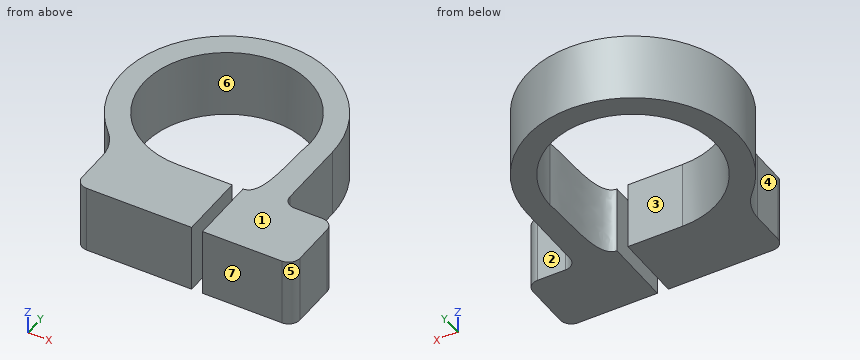
from build123d import *

# Parameters (mm, degrees)
F1_DEPTH = 9.525


with BuildPart() as f1:
    # F0 (on Top) → F1 (new body)
    with BuildSketch(Plane.XY):
        with BuildLine():
            ThreePointArc((0, -11.58875), (-8.194484, 8.194484), (11.58875, 0))
            add(Edge.make_bspline(
                [(9.147086, -11.58875), (12.021219, -11.58875), (11.099955, -3.330184), (11.58875, 0)],
                knots=[0, 0, 0, 0, 11.843177, 11.843177, 11.843177, 11.843177], degree=3))
            Line((9.147086, -11.58875), (9.147086, -21.11375))
            Line((9.147086, -21.11375), (20.259586, -21.11375))
            ThreePointArc((20.259586, -21.11375), (21.382118, -20.648782), (21.847086, -19.52625))
            Line((21.847086, -19.52625), (21.847086, -13.17625))
            ThreePointArc((21.847086, -13.17625), (21.382118, -12.053718), (20.259586, -11.58875))
            Line((20.259586, -11.58875), (16.35125, -11.58875))
            ThreePointArc((16.35125, -11.58875), (15.228718, -11.123782), (14.76375, -10.00125))
            Line((14.76375, -10.00125), (14.76375, 0))
            ThreePointArc((14.76375, 0), (-5.649843, 13.639926), (-10.439548, -10.439548))
            ThreePointArc((-10.439548, -10.439548), (-9.113907, -12.423509), (-8.648405, -14.76375))
            Line((-8.648405, -14.76375), (-8.648405, -19.52625))
            ThreePointArc((-8.648405, -19.52625), (-8.183437, -20.648782), (-7.060905, -21.11375))
            Line((-7.060905, -21.11375), (7.620076, -21.11375))
            Line((7.620076, -21.11375), (7.620076, -11.58875))
            Line((7.620076, -11.58875), (0, -11.58875))
        make_face()
    extrude(amount=F1_DEPTH)


solid = f1.part
Input: part model. Units: mm. Frame: model coordinates. Face numbers are marked on the shaded views. A direction names the side the tool comes from. Coordinates: 2 decimals unless noted, no trailing zeros. Loops run counter-clockwise (first coordinate to the right, second up) from the corner with the lowest first, then second, coordinate; pieces in that order, holes last.
(1) Section A-A on y = -17.5. Return the cut outline in (x, z) (3 decimals).
(2) Material intervals for probe 1 along Y at (x, z) = (0, 4.75); probe 2 along Y at (x, z) = (18, 3); probe 3 along Y at (x, z) = (5, 8), sorted ascending.
(3) Set-up query: the marked faces 1, 2, 3 and 4. Return all of +Z, -Z, +X, -X, +Y, -Y with unobstructed straight access to the full face (end or side cutting, diameter ignored); none if empty.
(4) First-contact query: pin 1 Ø1.5 at (x, z) = (0.5, 2) entering from +Y; pin 2 Ø2 at (y, z) = (11, 3) entering from +X; pin 3 Ø1 at (x, y) = (15, 3) entering from +Z; pin 4 Ø3 at (x, z) = (7.5, 5) entering from +Y. Flat tips, straight axial feed; report the tip coordinate or a pass-through.
(5) Section B-B on x = 4. Return the cut outline in (y, z) (3 decimals).
(6) Pull-direction query (X, two-part tool) for the marked faces 5, 6 and 7; classes: released by +X, released by -X, zero draft, split by the parting line, or undercut.
Data:
1. outline: (-8.648, 0) - (7.62, 0) - (7.62, 9.525) - (-8.648, 9.525) - close; (9.147, 0) - (21.847, 0) - (21.847, 9.525) - (9.147, 9.525) - close
2. probe 1: y = -21.11 to -11.59, 11.59 to 14.76
2. probe 2: y = -21.11 to -11.59
2. probe 3: y = -21.11 to -11.59, 10.45 to 13.89
3. face 1: +Z, +X, -X, +Y, -Y
3. face 2: +Z, -Z, +X, +Y
3. face 3: +Z, -Z
3. face 4: +Z, -Z, -X, -Y
4. pin 1: stops at y = 14.76
4. pin 2: stops at x = 10.86
4. pin 3: passes through
4. pin 4: stops at y = 13.49
5. outline: (-21.114, 0) - (-11.589, 0) - (-11.589, 9.525) - (-21.114, 9.525) - close; (10.877, 0) - (14.212, 0) - (14.212, 9.525) - (10.877, 9.525) - close
6. face 5: released by +X
6. face 6: undercut
6. face 7: zero draft
